Autodesk Inventor part; units mm, degrees
ref_plane "YZ Plane" through (0, 0, 0) normal (1, 0, 0) x (0, 1, 0)
ref_plane "XZ Plane" through (0, 0, 0) normal (0, 1, 0) x (-1, 0, 0)
ref_plane "XY Plane" through (0, 0, 0) normal (0, 0, 1) x (1, 0, 0)
sketch "Sketch1" plane through (0, 0, 0) normal (0, 0, 1) x (1, 0, 0)
  line L0 (-60.96, 57.15) -> (45.72, 57.15)
  line L1 (55.88, 46.99) -> (55.88, -46.99)
  line L2 (45.72, -57.15) -> (-60.96, -57.15)
  line L3 (-71.12, -46.99) -> (-71.12, 46.99)
  line L4 (-99.4659, 0) -> (84.2259, 0)
  line L5 (0, -82.9559) -> (0, 82.9559)
  arc A0 (-60.96, 57.15) -> (-71.12, 46.99) centre (-60.96, 46.99) ccw
  arc A1 (55.88, 46.99) -> (45.72, 57.15) centre (45.72, 46.99) ccw
  arc A2 (45.72, -57.15) -> (55.88, -46.99) centre (45.72, -46.99) ccw
  arc A3 (-71.12, -46.99) -> (-60.96, -57.15) centre (-60.96, -46.99) ccw
  circle A4 centre (0, 0) radius 40.64
  point P0 (55.88, -57.15)
  point P1 (55.88, 57.15)
  point P2 (-71.12, -57.15)
  point P3 (-71.12, 0)
  dimension "d0" = 127
  dimension "d1" = 114.3
  dimension "d2" = 55.88
  dimension "d3" = 10.16
  dimension "d6" = 81.28
extrude "Extrusion1" add sketch "Sketch1" along normal blind 157.48
extrude "Extrusion2" cut sketch "Sketch1" along normal blind 157.48 contours A4 L4 L5 | L5 L4 A4 | L5 A4 L4 | L4 A4 L5
sketch "Sketch2" plane through (0, 0, 157.48) normal (0, 0, 1) x (1, 0, 0)
  circle A0 centre (0, 0) radius 58.42 construction
  line L0 (0, 0) -> (45.72, 45.72) construction
  line L1 (0, 0) -> (64.6578, 0) construction
  circle A1 centre (41.3092, 41.3092) radius 8.89
  circle A2 centre (-41.3092, 41.3092) radius 8.89
  circle A3 centre (-41.3092, -41.3092) radius 8.89
  circle A4 centre (41.3092, -41.3092) radius 8.89
  dimension "d9" = 116.84
  dimension "d10" = 45
  dimension "d11" = 17.78
  dimension "d14" = 360
extrude "Extrusion3" cut sketch "Sketch2" against normal through all
sketch "Sketch3" plane through (0, 0, 157.48) normal (0, 0, 1) x (1, 0, 0)
  circle A0 centre (-60.96, 0) radius 5.08
  line L0 (-60.96, 5.08) -> (-31.75, 5.08)
  line L1 (-31.75, 5.08) -> (-31.75, -5.08)
  line L2 (-31.75, -5.08) -> (-60.96, -5.08)
  line L3 (-96.52, 0) -> (81.28, 0)
  point P0 (0, 0)
  point P1 (-31.75, 0)
  dimension "d18" = 10.16
  dimension "d19" = 60.96
  dimension "d20" = 10.16
extrude "Extrusion4" cut sketch "Sketch3" against normal through all contours L3 A0 | A0 L3
extrude "Extrusion5" cut sketch "Sketch3" against normal blind 5.08 contours L3 L1 L2 A0 | A0 L0 L1 L3
sketch "Sketch4" plane through (0, 0, 0) normal (0, 1, 0) x (-1, 0, 0)
  line L0 (45.72, 5.08) -> (-45.72, 5.08)
  line L1 (-45.72, 5.08) -> (-45.72, 0)
  line L2 (-45.72, 0) -> (45.72, 0)
  line L3 (45.72, 0) -> (45.72, 5.08)
  line L4 (0, -49.022) -> (0, 191.897)
  line L5 (-45.72, 0) -> (-55.88, 0)
  line L6 (60.96, 0) -> (-45.72, 0)
  line L7 (-45.72, 0) -> (-45.72, 157.48)
  line L8 (60.96, 157.48) -> (-45.72, 157.48)
  line L9 (60.96, 0) -> (60.96, 157.48)
  line L10 (40.64, 152.4) -> (55.88, 152.4)
  line L11 (55.88, 152.4) -> (55.88, 0)
  line L12 (55.88, 0) -> (40.64, 0)
  line L13 (40.64, 0) -> (40.64, 152.4)
  line L14 (71.12, 157.48) -> (71.12, 0)
  line L15 (71.12, 0) -> (66.04, 0)
  line L16 (66.04, 0) -> (66.04, 157.48)
  line L17 (66.04, 157.48) -> (71.12, 157.48)
  line L18 (-55.88, 0) -> (-55.88, 157.48)
  line L19 (-55.88, 157.48) -> (-40.64, 157.48)
  line L20 (-40.64, 157.48) -> (-40.64, 0)
  line L21 (-40.64, 0) -> (-55.88, 0)
  line L22 (45.72, 0) -> (96.52, 0)
  line L23 (96.52, 0) -> (96.52, 5.08)
  line L24 (96.52, 5.08) -> (45.72, 5.08)
  line L25 (45.72, 5.08) -> (45.72, 0)
  point P0 (0, 0)
  point P1 (0, 5.08)
  dimension "d25" = 91.44
  dimension "d26" = 5.08
  dimension "d27" = 50.8
revolve "Revolution1" cut sketch "Sketch4" angle 360 about axis through (0, 0, -10) along (0, 0, 1) contours L24 L11 L6 L3 | L24 L9 L6 L11 | L24 L16 L22 L9 | L24 L14 L15 L16 | L24 L23 L22 L14
ref_plane "Work Plane1" through (0, 0, 144.78) normal (0, 0, 1) x (1, 0, 0)
sketch "Sketch5" plane through (0, 0, 144.78) normal (0, 0, 1) x (1, 0, 0)
  arc A0 (-60.96, 57.15) -> (-71.12, 46.99) centre (-60.96, 46.99) ccw
  line L0 (-60.96, 57.15) -> (45.72, 57.15)
  arc A1 (55.88, 46.99) -> (45.72, 57.15) centre (45.72, 46.99) ccw
  line L1 (55.88, 46.99) -> (55.88, -46.99)
  arc A2 (45.72, -57.15) -> (55.88, -46.99) centre (45.72, -46.99) ccw
  line L2 (45.72, -57.15) -> (-60.96, -57.15)
  arc A3 (-71.12, -46.99) -> (-60.96, -57.15) centre (-60.96, -46.99) ccw
  line L3 (-71.12, -46.99) -> (-71.12, 46.99)
  circle A4 centre (-60.96, 0) radius 5.08
  circle A5 centre (41.3092, -41.3092) radius 8.89
  circle A6 centre (-41.3092, -41.3092) radius 8.89
  circle A7 centre (41.3092, 41.3092) radius 8.89
  circle A8 centre (-41.3092, 41.3092) radius 8.89
  circle A9 centre (0, 0) radius 40.64
sketch "Sketch6" plane through (0, 0, 144.78) normal (0, 0, 1) x (1, 0, 0)
  arc A0 (55.88, 33.6969) -> (55.88, -33.6969) centre (106.68, 0) ccw
  line L0 (55.88, -46.99) -> (55.88, 46.99)
  arc A1 (-33.6969, 57.15) -> (33.6969, 57.15) centre (0, 107.95) ccw
  line L1 (45.72, 57.15) -> (-60.96, 57.15)
  arc A2 (33.6969, -57.15) -> (-33.6969, -57.15) centre (0, -107.95) ccw
  line L2 (-60.96, -57.15) -> (45.72, -57.15)
  line L3 (-40.3212, -5.08) -> (-60.96, -5.08)
  arc A3 (-60.96, 5.08) -> (-60.96, -5.08) centre (-60.96, 0) ccw
  line L4 (-60.96, 5.08) -> (-40.3212, 5.08)
  arc A4 (-40.3212, -5.08) -> (-40.3212, 5.08) centre (0, 0) ccw
  circle A5 centre (41.3092, -41.3092) radius 8.89
  circle A6 centre (-41.3092, -41.3092) radius 8.89
  circle A7 centre (41.3092, 41.3092) radius 8.89
  circle A8 centre (-41.3092, 41.3092) radius 8.89
  line L5 (55.88, -46.99) -> (55.88, 46.99)
  arc A9 (55.88, 46.99) -> (45.72, 57.15) centre (45.72, 46.99) ccw
  line L6 (45.72, 57.15) -> (-60.96, 57.15)
  arc A10 (-60.96, 57.15) -> (-71.12, 46.99) centre (-60.96, 46.99) ccw
  line L7 (-71.12, 46.99) -> (-71.12, -46.99)
  arc A11 (-71.12, -46.99) -> (-60.96, -57.15) centre (-60.96, -46.99) ccw
  line L8 (-60.96, -57.15) -> (45.72, -57.15)
  arc A12 (45.72, -57.15) -> (55.88, -46.99) centre (45.72, -46.99) ccw
  arc A13 (-60.96, 57.15) -> (-71.12, 46.99) centre (-60.96, 46.99) ccw
  line L9 (-60.96, 57.15) -> (45.72, 57.15)
  arc A14 (55.88, 46.99) -> (45.72, 57.15) centre (45.72, 46.99) ccw
  line L10 (55.88, 46.99) -> (55.88, -46.99)
  arc A15 (45.72, -57.15) -> (55.88, -46.99) centre (45.72, -46.99) ccw
  line L11 (45.72, -57.15) -> (-60.96, -57.15)
  arc A16 (-71.12, -46.99) -> (-60.96, -57.15) centre (-60.96, -46.99) ccw
  line L12 (-71.12, -46.99) -> (-71.12, 46.99)
  circle A17 centre (-60.96, 0) radius 5.08
  circle A18 centre (41.3092, -41.3092) radius 8.89
  circle A19 centre (-41.3092, -41.3092) radius 8.89
  circle A20 centre (41.3092, 41.3092) radius 8.89
  circle A21 centre (-41.3092, 41.3092) radius 8.89
  circle A22 centre (0, 0) radius 40.64
  dimension "d32" = 121.92
  dimension "d33" = 50.8
  dimension "d34" = 121.92
  dimension "d35" = 50.8
  dimension "d36" = 121.92
  dimension "d37" = 50.8
extrude "Extrusion6" cut sketch "Sketch6" against normal blind 5.08 contours L0 A0 | A1 L1 | L2 A2
pattern_linear "Rectangular Pattern1" count 9 spacing 15.24 along (0, 0, -1) of "Extrusion6"
equation "\"BendRadius\" = Thickness"
equation "\"BendReliefWidth\" = Thickness"
equation "\"BendReliefDepth\" = 0.5 * Thickness"
equation "\"CornerReliefSize\" = 4 * Thickness"
equation "\"MinimumRemnant\" = 2 * Thickness"
equation "\"TransitionRadius\" = BendRadius"
equation "\"JacobiRadiusSize\" = BendRadius"
equation "\"GapSize\" = Thickness"
properties part number "cylinder" material "Aluminum 6061"
Model file for the job. Use its own axes, mm. A direction names the side the tool comes from. Give positions to 0.01 mm unless a question says otherwise; leave off trailing zeros. Order: outer loops, then holes, each group sorted by start corner. A loop starts at its lowest first (then second) coordinate and runs counter-clockwise, first axis right, second up. Notation, with made-up numbers: M 1,76 L 42,76 A22 ccw 42,85 Z; hole C -33.5,67 d2. An arc over 180 degrees is marked long. Put each result on its own line as item: value. Start each with the question number.
(1) Tool access for faces 4 (the face through (-50, -5.08, 155)), 5 (the face through (45.722, 0.5, 66.076)), 6 (the face through (0, 53, 114.3)): list every direction of +Z, -Z, +X, -X, +Y, -Y with a clear straight run to the whole face (end or side of a thin tool).
(2) Band-saw the part on B-B on z = 91. Give the cut face in (x, y).
(3) Band-saw the part on C-C on x = -43. Give the cut face in (y, z), then the cut area to 3 significant figures.
(4) Pin check, flat tip, straight feed: pin 1 Ø11 at (x, y) = (50, 14.5) entering from -Z. Stop position of the tip, or through.
(5) Pull direction Z, two halves, no side cores. Call faces 1 (the face through (-43.61, -13.73, 2.58)), 2 (the face through (-48, 0, 152.4)), 3 (the face through (52, 0, 53.34)): released by +Z, released by -Z, zero draft, split by the parting line, or undercut.
(6) Drill centre lines: L1, parallel to X at y = 0, z = 60.5; L2, parallel to X at y = 2, z = 64; L3, parallel to Y at x = 45, z = 107.5. Where is each one in solid material? Low to high. Write a range as [from, to].
(7) Band-saw the part on A-A on y = 0. Count the separate pieces of the cut face and the enclosed holes in it, then the cut area to 3 significant figures.
Results below:
1. face 4: +Z
1. face 5: +X
1. face 6: +Y
2. outline: M -71.12,-46.99 A10.16 ccw -60.96,-57.15 L 45.72,-57.15 A10.16 ccw 55.88,-46.99 L 55.88,46.99 A10.16 ccw 45.72,57.15 L -60.96,57.15 A10.16 ccw -71.12,46.99 Z; hole C -60.96,0 d10.16; hole C -41.31,-41.31 d17.78; hole C -41.31,41.31 d17.78; hole C 0,0 d81.28; hole C 41.31,-41.31 d17.78; hole C 41.31,41.31 d17.78
3. outline: M -57.15,5.08 L -50.04,5.08 L -50.04,157.48 L -57.15,157.48 Z; M -32.58,5.08 L -15.53,5.08 L -15.53,0 L 15.53,0 L 15.53,5.08 L 32.58,5.08 L 32.58,157.48 L 5.08,157.48 L 5.08,152.4 L -5.08,152.4 L -5.08,157.48 L -32.58,157.48 Z; M 50.04,5.08 L 57.15,5.08 L 57.15,157.48 L 50.04,157.48 Z
3. area: 12,200 mm2
4. pin 1: stops at z = 5.08
5. face 1: zero draft
5. face 2: released by +Z
5. face 3: undercut
6. L1: x = [-71.12, -66.04], [-55.88, -40.64], [40.64, 55.88]
6. L2: x = [-71.12, -65.63], [-56.29, -40.59], [40.59, 45.75]
6. L3: y = [-57.15, -49.4], [-33.22, 33.22], [49.4, 57.15]
7. separate pieces: 3
7. enclosed holes: 0
7. area: 4,930 mm2
